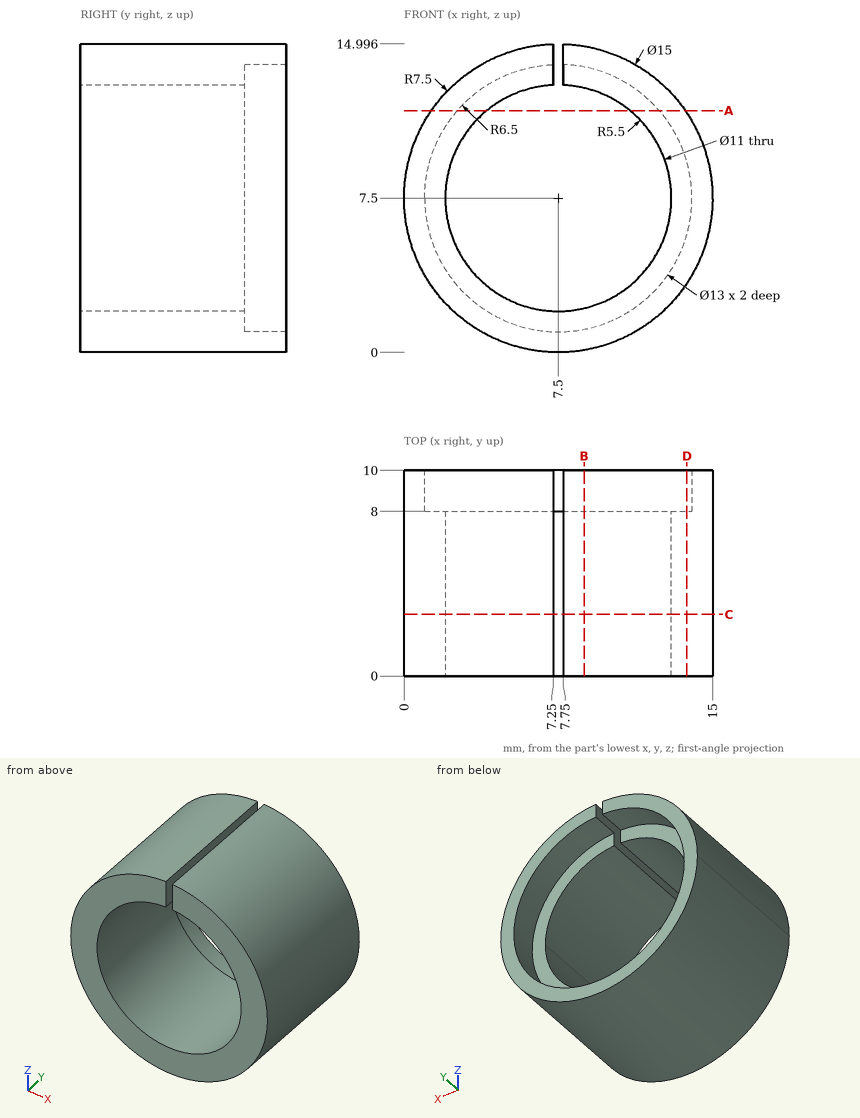
Input: dimensioned drawing with shaded views. Units: mm. Origin: part minimum x, y, z. Round coordinates to 2 decimals unless told otherwise and drop trailing zeros. Order: outer loops, then holes, each group sorted by start corner. A loop starts at its lowest first (then second) coordinate and runs counter-clockwise, first axis right, second up. Notation, with made-up numbers: (18.5, 4.25) - (38.5, 4.25) arc R21 cw to (38.5, 11.25) - close; hole circle Ø4 at (56.25, 29). An arc over 180 degrees is marked (long way). Use CSV: the item, a comma, the result in double quotes. Start each with the question number.
Q1. Section query B-B (x = 8.75). Return loops of the section in (y, z) (1 decimal), and give its area (3 significant figures).
Q2. Material intervals for line 1 along X through (y, z) = (9.2, 7.5); line 2 along X through (y, z) = (3.75, 7.5); line 3 along Z through (x, y) = (7.5, 2.25), sorted ascending. Write a range as from..to.
Q3. First-contact query: pin 1 (1.5 mm diameter, centred on y = 6, z = 9.5, fed in from -X) (3 decimals); pin 2 (3 mm diameter, centred on y = 6, z = 1.5, fed in from +X); pin 3 (1.5 mm diameter, centred on y = 2.5, z = 13, fed in from -X). Flat tips, straight axial feed; report the tip coordinate or a pass-through.
Q4. Section query D-D (x = 13.75). Return loops of the section in (y, z).
Q5. Section query A-A (z = 11.75). Return loops of the section in (x, y).
Q6. Section query C-C (y = 3). Return loops of the section in (x, z), and give its area (3 significant figures).
Result set:
1,outline,"(0, 0.1) - (10, 0.1) - (10, 1.1) - (8, 1.1) - (8, 2.1) - (0, 2.1) - close; (0, 12.9) - (8, 12.9) - (8, 13.9) - (10, 13.9) - (10, 14.9) - (0, 14.9) - close"
1,area,"36.7 mm2"
2,line 1,"x = 0..1, 14..15"
2,line 2,"x = 0..2, 13..15"
2,line 3,"z = 0..2"
3,pin 1,"stops at x = 0.105"
3,pin 2,"stops at x = 13.5"
3,pin 3,"stops at x = 1.7"
4,outline,"(0, 3.35) - (10, 3.35) - (10, 5.71) - (8, 5.71) - (8, 9.29) - (10, 9.29) - (10, 11.65) - (0, 11.65) - close"
5,outline,"(1.32, 0) - (4.01, 0) - (4.01, 8) - (2.58, 8) - (2.58, 10) - (1.32, 10) - close; (10.99, 0) - (13.68, 0) - (13.68, 10) - (12.42, 10) - (12.42, 8) - (10.99, 8) - close"
6,outline,"(7.25, 12.99) - (7.25, 15) arc R7.5 ccw (long way) to (7.75, 15) - (7.75, 12.99) arc R5.5 cw (long way) to start"
6,area,"80.7 mm2"
